Geometry: see drawing. Coordinates: mm, zero at the bounding-box minimum. A direction names the side the tool comes from. Give positions to 0.01 mm unless a question says otherwise; leave off trailing zeros. Write each loop counter-clockwise with the first axis right and the second up, starting at its lowest first coordinate (ties: lowest second). Pieces come first, ordered by that corner, then holes.
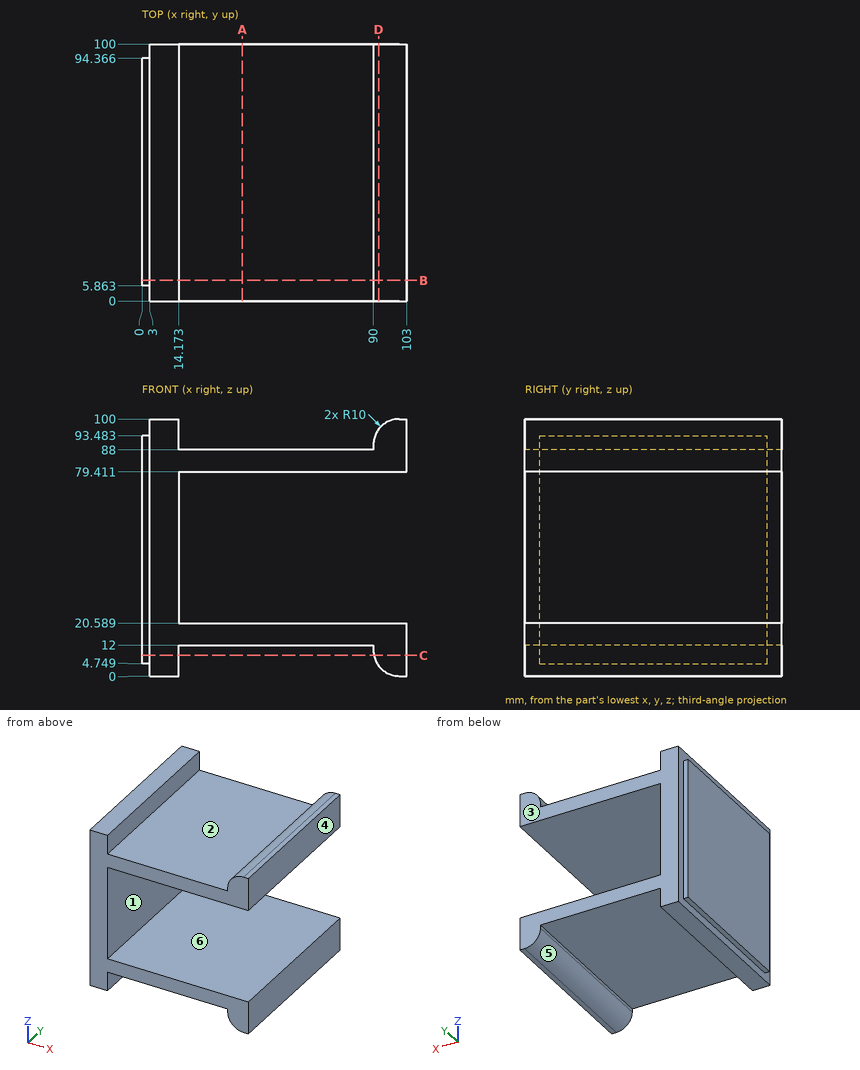
1. Pull-direction query (Z, two-part tool) for the marked faces 1, 2 and 3; classes: pulls with the +Z half, pulls with the -Z half, needs draft (parallel to the pull), parting line crosses it, or undercut.
2. Access query for the marked faces 4, 5 and 6. Directions: +Z, -Z, +X, -X, +Y, -Y. A direction counts if a zero-diameter tool reaches every point of the face in a straight line with its end or side. Return the directions, or none.
3. Section query D-D (x = 92). Return loops of the section in (y, z).
4. Line query: probe 1 along Z at (x, y) = (18, 45.5); probe 2 along X at (y, z) = (63, 55); probe 3 along X at (y, z) = (56.5, 5). Output: solid intervals per line, ascending.
5. Section query B-B (y = 8). Return loops of the section in (x, z), plus the area to 3 significant figures.
6. Section query A-A (x = 39). Return loops of the section in (y, z).
7. Pin query (flat end, axial travel): P1, Ø2, axis at y = 86.5, z = 34, coming from the -X side; P2, Ø3, axis at y = 22, z = 44.5, coming from the +X side; P3, Ø2.5, axis at x = 1.5, y = 56, coming from the +Z side; P4, Ø12, axis at x = 57, y = 85.5, coming from the -Z side. Return the tip coordinate at first contact, or that it passes through.
8. Section query C-C (z = 8). Return loops of the section in (x, y).
The answers:
1. face 1: undercut
1. face 2: pulls with the +Z half
1. face 3: needs draft
2. face 4: +Z, -Z, +X, +Y, -Y
2. face 5: -Z, +Y, -Y
2. face 6: +X, +Y, -Y
3. outline: (0, 4) - (100, 4) - (100, 20.59) - (0, 20.59) - close; (0, 79.41) - (100, 79.41) - (100, 96) - (0, 96) - close
4. probe 1: z = 12 to 20.59, 79.41 to 88
4. probe 2: x = 0 to 14.17
4. probe 3: x = 0 to 14.17, 91.34 to 103
5. outline: (0, 4.75) - (3, 4.75) - (3, 0) - (14.17, 0) - (14.17, 12) - (90, 12) - (90, 10) arc R10 ccw to (100, 0) - (103, 0) - (103, 20.59) - (14.17, 20.59) - (14.17, 79.41) - (103, 79.41) - (103, 100) - (100, 100) arc R10 ccw to (90, 90) - (90, 88) - (14.17, 88) - (14.17, 100) - (3, 100) - (3, 93.48) - (0, 93.48) - close
5. area: 3,180 mm2
6. outline: (0, 12) - (100, 12) - (100, 20.59) - (0, 20.59) - close; (0, 79.41) - (100, 79.41) - (100, 88) - (0, 88) - close
7. P1: stops at x = 0
7. P2: stops at x = 14.17
7. P3: stops at z = 93.48
7. P4: stops at z = 12
8. outline: (0, 5.86) - (3, 5.86) - (3, 0) - (14.17, 0) - (14.17, 100) - (3, 100) - (3, 94.37) - (0, 94.37) - close; (90.2, 0) - (103, 0) - (103, 100) - (90.2, 100) - close
